```python
from build123d import *

# Parameters (mm, degrees)
F0_R     = 2.75
F1_DEPTH = 18
F2_R     = 6
F3_DEPTH = 7.5005674408


# Not quite as in the source:
# - a feature names something its author has since deleted; it is built from what else it names


with BuildPart() as f1:
    # F0 (on Top) → F1 (new body)
    with BuildSketch(Plane.XY):
        with BuildLine():
            ThreePointArc((-14.8575540239, 3.74907491), (-12.2599082251, 2.6220374098), (-11.1908445954, 0))
            Line((-11.1908445954, 0), (12.8071008226, 0))
            ThreePointArc((12.8071008226, 0), (13.8537114507, 2.599708945), (16.4096532115, 3.74907491))
            Line((16.4096532115, 3.74907491), (-14.8575540239, 3.74907491))
        make_face()
        with BuildLine():
            ThreePointArc((-14.8838884093, -3.7495674408), (-12.269133, -2.6314363285), (-11.1908445954, 0))
            ThreePointArc((-11.1908445954, 0), (-12.2599082251, 2.6220374098), (-14.8575540239, 3.74907491))
            ThreePointArc((-14.8575540239, 3.74907491), (-18.6901888916, 0.0701238113), (-14.9978007816, -3.7495674408))
            Line((-14.9978007816, -3.7495674408), (-14.8838884093, -3.7495674408))
        make_face()
        with Locations((-14.9408445954, 0)):
            Circle(F0_R, mode=Mode.SUBTRACT)
        with BuildLine():
            ThreePointArc((16.4096532115, 3.74907491), (13.8537114507, 2.599708945), (12.8071008226, 0))
            ThreePointArc((12.8071008226, 0), (13.858191018, -2.60436268), (16.4225626025, -3.7495674408))
            ThreePointArc((16.4225626025, -3.7495674408), (19.1635180845, -2.7009643866), (20.3112099866, 0))
            ThreePointArc((20.3112099866, 0), (19.2645993584, 2.599708945), (16.7086575976, 3.74907491))
            Line((16.7086575976, 3.74907491), (16.4096532115, 3.74907491))
        make_face()
        with Locations((16.5591554046, 0)):
            Circle(F0_R, mode=Mode.SUBTRACT)
        with BuildLine():
            Line((12.8071008226, 0), (-11.1908445954, 0))
            ThreePointArc((-11.1908445954, 0), (-12.269133, -2.6314363285), (-14.8838884093, -3.7495674408))
            Line((-14.8838884093, -3.7495674408), (16.4225626025, -3.7495674408))
            ThreePointArc((16.4225626025, -3.7495674408), (13.858191018, -2.60436268), (12.8071008226, 0))
        make_face()
    extrude(amount=F1_DEPTH)

    # F2 (on face) → F3 (cut, through all)
    with BuildSketch(Plane.XZ.offset(3.7495674408)):
        with Locations((0.0021992184, 9)):
            Circle(F2_R)
    extrude(amount=-F3_DEPTH, mode=Mode.SUBTRACT)


solid = f1.part
```
Can you work these out from the model? Positions are in its coordinate system, mm. Coordinates: 2 decimals unless noted, no trailing zeros. Loops run counter-clockwise (first coordinate to the right, second up) from the corner with the lowest first, then second, coordinate; pieces in that order, holes last. Notation, with made-up numbers: (-8, 57) - (20, 57) arc R31 cw to (20, 89) - close; hole circle Ø4 at (-1, 64.5). An arc over 180 degrees is marked (long way). Use a Markdown table: item, result.
Item 1: If I drill on probe 1 along X at (y, z) = (1.75, 5.5); probe 2 along X at (y, z) = (-0.75, 14.5); probe 3 along X at (y, z) = (1.5, 15.75), over which ranges is the centre line in solid material (lowest first)? Write a range as from..to.
Numbers:
| item | result |
|---|---|
| probe 1 | x = -18.26..-17.06, -12.82..-4.87, 4.88..14.44, 18.68..19.88 |
| probe 2 | x = -18.62..-17.59, -12.3..-2.4, 2.4..13.91, 19.2..20.24 |
| probe 3 | x = -18.38..-17.25, -12.64..14.25, 18.86..20 |
Item 2: I want a section at B-B on y = 1. Please give me the cut outline in (x, z).
Numbers:
| item | result |
|---|---|
| outline | (-18.56, 0) - (-17.5, 0) - (-17.5, 18) - (-18.56, 18) - close; (-12.38, 0) - (14, 0) - (14, 18) - (-12.38, 18) - close; (19.12, 0) - (20.18, 0) - (20.18, 18) - (19.12, 18) - close; hole circle Ø12 at (0, 9) |
Item 3: Will these pins go through, and if not, where does the flat tip stop? pin 1 (6 mm diameter, centred on x = -9, z = 2.5, fed in from -Y); pin 2 (9.5 mm diameter, centred on x = 0, z = 9, fed in from -Y).
Numbers:
| item | result |
|---|---|
| pin 1 | stops at y = -3.75 |
| pin 2 | passes through |
Item 4: We'd pull the mould along Z, two halves only. Please class faces 1 (the face through (-1.298, -0.053, 3.143)), 2 (the face through (1, 0, 18)), 3 (the face through (13.81, 0.12, 8.87)), 4 (the face through (1, 0, 0)): released by +Z, released by -Z, zero draft, split by the parting line, or undercut.
Numbers:
| item | result |
|---|---|
| face 1 | undercut |
| face 2 | released by +Z |
| face 3 | zero draft |
| face 4 | released by -Z |
Item 5: I want a section at A-A on z = 9. Please give me the cut outline in (x, y).
Numbers:
| item | result |
|---|---|
| outline | (-15, -3.75) - (-6, -3.75) - (-6, 3.75) - (-14.86, 3.75) arc R3.75 ccw (long way) to start; (6, -3.75) - (16.42, -3.75) arc R3.75 ccw to (16.71, 3.75) - (6, 3.75) - close; hole circle Ø5.5 at (-14.94, 0); hole circle Ø5.5 at (16.56, 0) |
Item 6: I want a section at D-D on z = 1.5. Please give me the cut outline in (x, y), and give its area (3 significant figures).
Numbers:
| item | result |
|---|---|
| outline | (-15, -3.75) - (16.42, -3.75) arc R3.75 ccw to (16.71, 3.75) - (-14.86, 3.75) arc R3.75 ccw (long way) to start; hole circle Ø5.5 at (-14.94, 0); hole circle Ø5.5 at (16.56, 0) |
| area | 233 mm2 |
Item 7: I want a section at C-C on x = 5.5. Please give me the cut outline in (y, z), and give its area (3 significant figures).
Numbers:
| item | result |
|---|---|
| outline | (-3.75, 0) - (3.75, 0) - (3.75, 6.6) - (-3.75, 6.6) - close; (-3.75, 11.4) - (3.75, 11.4) - (3.75, 18) - (-3.75, 18) - close |
| area | 98.9 mm2 |
